from build123d import *

# Parameters (mm, degrees)
SKETCH_W        = 25
SKETCH_H        = 24
PAD_DEPTH       = 1.75
SKETCH001_R     = 1
POCKET_DEPTH    = 1.75
SKETCH002_W     = 8
SKETCH002_H     = 8
PAD001_DEPTH    = 3
SKETCH003_R     = 3.75
PAD002_DEPTH    = 1.5
SKETCH004_R     = 1
POCKET001_DEPTH = 1
PAD003_DEPTH    = 1.25


with BuildPart() as part:
    # Sketch → Pad (new body)
    with BuildSketch(Plane.XY):
        Rectangle(SKETCH_W, SKETCH_H)
    extrude(amount=PAD_DEPTH)

    # Sketch001 (on Face6 of Pad) → Pocket (cut)
    with BuildSketch(Plane.XY.offset(1.75)):
        with Locations((-10.5, 10)):
            Circle(SKETCH001_R)
        with Locations((10.5, 10)):
            Circle(SKETCH001_R)
        with Locations((-10.5, -2.5)):
            Circle(SKETCH001_R)
        with Locations((10.5, -2.5)):
            Circle(SKETCH001_R)
    extrude(amount=-POCKET_DEPTH, mode=Mode.SUBTRACT)

    # Sketch002 (on Face5 of Pocket) → Pad001 (join)
    with BuildSketch(Plane.XY.offset(1.75)):
        with Locations((0, -2.5)):
            Rectangle(SKETCH002_W, SKETCH002_H)
    extrude(amount=PAD001_DEPTH)

    # Sketch003 (on Face15 of Pad001) → Pad002 (join)
    with BuildSketch(Plane.XY.offset(4.75)):
        with Locations((0, -2.5)):
            Circle(SKETCH003_R)
    extrude(amount=PAD002_DEPTH)

    # Sketch004 (on Face17 of Pad002) → Pocket001 (cut)
    with BuildSketch(Plane.XY.offset(6.25)):
        with Locations((0, -2.5)):
            Circle(SKETCH004_R)
    extrude(amount=-POCKET001_DEPTH, mode=Mode.SUBTRACT)

    # Sketch005 (on Face5 of Pocket001) → Pad003 (join)
    with BuildSketch(Plane.XY.offset(1.75)):
        Polygon((-3.75, 12), (-3.75, 7), (-2.75, 7), (-2.75, 1.5), (2.75, 1.5), (2.75, 7), (3.75, 7), (3.75, 12), align=None)
    extrude(amount=PAD003_DEPTH)


solid = part.part
Source: CAD feature listing. Evaluate the final solid. Frame: model axes, mm. A direction names the side the tool comes from. Coordinates: 2 decimals unless noted, no trailing zeros. Loops run counter-clockwise (first coordinate to the right, second up) from the corner with the lowest first, then second, coordinate; pieces in that order, holes last. Notation, with made-up numbers: M -22,80 L -10,80 A21 ccw -10,108 Z; hole C -16.75,45 d2. An arc over 180 degrees is marked long. Answer in a Markdown table with one row per item.
Q1. Section A-A on y = -2.5. Return the cut outline in (x, z).
Answers below:
| item | result |
|---|---|
| outline | M -12.5,0 L -11.5,0 L -11.5,1.75 L -12.5,1.75 Z; M -9.5,0 L 9.5,0 L 9.5,1.75 L 4,1.75 L 4,4.75 L 3.75,4.75 L 3.75,6.25 L 1,6.25 L 1,5.25 L -1,5.25 L -1,6.25 L -3.75,6.25 L -3.75,4.75 L -4,4.75 L -4,1.75 L -9.5,1.75 Z; M 11.5,0 L 12.5,0 L 12.5,1.75 L 11.5,1.75 Z |
Q2. Ray query, probe 1 along Y at (x, z) = (10.5, 0.95); probe 2 along Y at (x, z) = (0, 6); probe 3 along Y at (x, z) = (-3.25, 4). Return the intervals inside material, ascending. Write a range as from..to.
Answers below:
| item | result |
|---|---|
| probe 1 | y = -12..-3.5, -1.5..9, 11..12 |
| probe 2 | y = -6.25..-3.5, -1.5..1.25 |
| probe 3 | y = -6.5..1.5 |
Q3. Section D-D on y = 4.75. Return the cut outline in (x, z), plus the area to 3 significant figures.
Answers below:
| item | result |
|---|---|
| outline | M -12.5,0 L 12.5,0 L 12.5,1.75 L 2.75,1.75 L 2.75,3 L -2.75,3 L -2.75,1.75 L -12.5,1.75 Z |
| area | 50.6 mm^2 |
Q4. First-contact query: pin 1 (0.5 mm diameter, centred on x = -3.5, z = 2.5, fed in from -Y); pin 2 (1.4 mm diameter, centred on y = 9, z = 2.5, fed in from +X); pin 3 (2 mm diameter, centred on x = -0.5, y = 6.5, fed in from +Z); pin 4 (3 mm diameter, centred on x = -2, z = 3, fed in from -Y). Flat tips, straight axial feed; report the tip coordinate or a pass-through.
Answers below:
| item | result |
|---|---|
| pin 1 | stops at y = -6.5 |
| pin 2 | stops at x = 3.75 |
| pin 3 | stops at z = 3 |
| pin 4 | stops at y = -12 |
Q5. Draft query along X for faces 6 (the flat face through (0, -2, 5.25)), 7 (the flat face through (-12.5, 0, 1)), 8 (the cylindrical face through (-3.746, -2.335, 5.49)), 9 (the cylindrical face through (-10.63, 10.99, 0.89)). Return one class per face: pulls with the +X half, pulls with the -X half, needs draft (parallel to the pull), parting line crosses it, or undercut.
Answers below:
| item | result |
|---|---|
| face 6 | undercut |
| face 7 | pulls with the -X half |
| face 8 | parting line crosses it |
| face 9 | undercut |
Q6. Set-up query: faces 1 (the flat face through (-2.75, 4, 2)), 2 (the flat face through (-3.75, 10, 2)), 3 (the flat face through (0, -6.5, 3)), 4 (the flat face through (4, -3, 3)), 5 (the flat face through (3, 7, 2)). Return all of +Z, -Z, +X, -X, +Y, -Y with unobstructed straight access to the full face (end or side cutting, diameter ignored); none if empty.
Answers below:
| item | result |
|---|---|
| face 1 | +Z, -X |
| face 2 | +Z, -X, +Y |
| face 3 | +Z, +X, -X, -Y |
| face 4 | +Z, +X, +Y, -Y |
| face 5 | +Z, +X |
Q7. Section C-C on z = 0.75. Return the cut outline in (x, y).
Answers below:
| item | result |
|---|---|
| outline | M -12.5,-12 L 12.5,-12 L 12.5,12 L -12.5,12 Z; hole C -10.5,-2.5 d2; hole C -10.5,10 d2; hole C 10.5,-2.5 d2; hole C 10.5,10 d2 |
Q8. Section B-B on x = 10.5. Return the cut outline in (y, z).
Answers below:
| item | result |
|---|---|
| outline | M -12,0 L -3.5,0 L -3.5,1.75 L -12,1.75 Z; M -1.5,0 L 9,0 L 9,1.75 L -1.5,1.75 Z; M 11,0 L 12,0 L 12,1.75 L 11,1.75 Z |
